```python
from build123d import *

# Parameters (mm, degrees)
F0_R          = 25.4
F0_R_2        = 23.8125
F1_DEPTH      = 304.8
F3_R          = 3.81
F4_DEPTH      = 25.4
F4_DEPTH_BACK = 25.4


with BuildPart() as f1:
    # F0 (on Front) → F1 (new body)
    with BuildSketch(Plane.XZ):
        Circle(F0_R)
        Circle(F0_R_2, mode=Mode.SUBTRACT)
    extrude(amount=-F1_DEPTH)

    # F3 (on Top) → F4 (cut, two sides)
    with BuildSketch(Plane.XY) as f4_sk:
        with Locations((0, 19.05)):
            Circle(F3_R)
        with Locations((0, 285.75)):
            Circle(F3_R)
        with Locations((0, 38.1)):
            Circle(F3_R)
    extrude(amount=F4_DEPTH, mode=Mode.SUBTRACT)
    extrude(f4_sk.sketch, amount=-F4_DEPTH_BACK, mode=Mode.SUBTRACT)


solid = f1.part
```
Could you check a few things on this model? Use its own coordinates, in mm. Coordinates: 2 decimals unless noted, no trailing zeros. Write each loop counter-clockwise with the first axis right and the second up, starting at its lowest first coordinate (ties: lowest second). Pieces come first, ordered by that corner, then holes. Notation, with made-up numbers: (76.25, 6) -> (85.25, 6) arc R27 ccw to (85.25, 39) -> close; hole circle Ø8 at (-11, 16). An arc over 180 degrees is marked (long way). Return JSON: item names as keys, results as strings.
(1) Imagine slicing it at C-C, the plane z = 0. Please give me the cut outline in (x, y).
Numbers:
{"outline": "(-25.4, 0) -> (-23.81, 0) -> (-23.81, 304.8) -> (-25.4, 304.8) -> close; (23.81, 0) -> (25.4, 0) -> (25.4, 304.8) -> (23.81, 304.8) -> close"}
(2) I need wall thicknesses on L1, parallel to Y at x = 0, z = 24.8; L2, parallel to Z at x = 0, y = 192; L3, parallel to X at y = 137.5, z = 1.5. Which ranges of each line are inside material? Lowest first, please.
Numbers:
{"L1": "y = 0 to 15.24, 22.86 to 34.29, 41.91 to 281.94, 289.56 to 304.8", "L2": "z = -25.4 to -23.81, 23.81 to 25.4", "L3": "x = -25.36 to -23.77, 23.77 to 25.36"}
(3) Imagine slicing it at B-B, the plane y = 19.05. Please give me the cut outline in (x, z) (1 decimal).
Numbers:
{"outline": "(-3.8, -25.1) -> (-3.8, -23.5) arc R23.8 cw to (-3.8, 23.5) -> (-3.8, 25.1) arc R25.4 ccw to start; (3.8, -25.1) arc R25.4 ccw to (3.8, 25.1) -> (3.8, 23.5) arc R23.8 cw to (3.8, -23.5) -> close"}
(4) Imagine slicing it at A-A, the plane x = 0. Count the separate pieces of the cut face and the enclosed holes in it, then the cut area to 3 significant figures.
Numbers:
{"separate pieces": "8", "enclosed holes": "0", "area": "895 mm2"}
(5) I'm going to push flat-ended pins straight in: pin 1 (12 mm diameter, centred on x = -3, y = 132.5, fed in from -Z); pin 2 (10 mm diameter, centred on y = 102.5, z = 19.5, fed in from +X); pin 3 (6 mm diameter, centred on x = -11, y = 180, fed in from +Z); pin 4 (10 mm diameter, centred on x = -17, y = 214, fed in from +Z). Where does each tip first touch, or does it pass through?
Numbers:
{"pin 1": "stops at z = -25.4", "pin 2": "stops at x = 20.85", "pin 3": "stops at z = 24.11", "pin 4": "stops at z = 22.39"}
(6) Imagine slicing it at D-D, the plane y = 240. Please give me the cut outline in (x, z) (1 decimal).
Numbers:
{"outline": "circle Ø50.8 at (0, 0); hole circle Ø47.6 at (0, 0)"}
(7) We'd pull the mould along X, two halves only. Please class faces 1 (the cylindrical face through (-5.506, 150.266, -24.796)), 2 (the cylindrical face through (3.52, 36.64, 24.43)), 3 (the flat face through (-23, 304.8, -7)): +X half, -X half, draft (parallel to the pull), parting line (faces both ways), or undercut.
Numbers:
{"face 1": "parting line", "face 2": "undercut", "face 3": "draft"}
